from build123d import *

# Parameters (mm, degrees)
SKETCH1_W                 = 58.4
SKETCH1_H                 = 36.8
BOSS_EXTRUDE1_DEPTH       = 12.7
SKETCH2_R                 = 0.5
SKETCH2_R_2               = 0.75
SKETCH2_R_3               = 0.25
BOSS_EXTRUDE2_DEPTH       = 4.3
M3X0_5_TAPPED_HOLE1_D     = 2.5
M3X0_5_TAPPED_HOLE1_DEPTH = 4.5
M3X0_5_TAPPED_HOLE1_TIP   = 0.751075774
SKETCH6_R                 = 1.5
BOSS_EXTRUDE3_DEPTH       = 0.01


with BuildPart() as part:
    # Sketch1 → Boss-Extrude1 (new body)
    with BuildSketch(Plane(origin=(0, 0, 0), x_dir=(1, 0, 0), z_dir=(0, 1, 0))):
        Rectangle(SKETCH1_W, SKETCH1_H)
    extrude(amount=BOSS_EXTRUDE1_DEPTH)

    # Sketch2 → Boss-Extrude2 (add)
    with BuildSketch(Plane.XZ):
        with Locations((-25.4, 0)):
            Circle(SKETCH2_R)
        with Locations((-25.4, 3.81)):
            Circle(SKETCH2_R)
        with Locations((-25.4, 7.62)):
            Circle(SKETCH2_R)
        with Locations((-25.4, -7.62)):
            Circle(SKETCH2_R)
        with Locations((25.4, 7.62)):
            Circle(SKETCH2_R_2)
        with Locations((25.4, 3.81)):
            Circle(SKETCH2_R)
        with Locations((25.4, 0)):
            Circle(SKETCH2_R)
        with Locations((25.4, -3.81)):
            Circle(SKETCH2_R)
        with Locations((25.4, -7.62)):
            Circle(SKETCH2_R_2)
        with Locations((27.94, 0)):
            Circle(SKETCH2_R_3)
        with Locations((27.94, -2)):
            Circle(SKETCH2_R_3)
        with Locations((27.94, -4)):
            Circle(SKETCH2_R_3)
        with Locations((27.94, -6)):
            Circle(SKETCH2_R_3)
        with Locations((27.94, 2)):
            Circle(SKETCH2_R_3)
        with Locations((27.94, 4)):
            Circle(SKETCH2_R_3)
        with Locations((27.94, 6)):
            Circle(SKETCH2_R_3)
    extrude(amount=BOSS_EXTRUDE2_DEPTH)

    # M3x0.5 Tapped Hole1
    with Locations(Plane(origin=(-23.6, 12.7, -13.06), x_dir=(0, 0, 1), z_dir=(0, 1, 0))):
        with Locations((0, 0), (26.16, 0), (26.16, 47.24)):
            Hole(M3X0_5_TAPPED_HOLE1_D / 2, depth=M3X0_5_TAPPED_HOLE1_DEPTH)
            with Locations((0, 0, -(M3X0_5_TAPPED_HOLE1_DEPTH + M3X0_5_TAPPED_HOLE1_TIP / 2))):  # 118° drill point
                Cone(0, M3X0_5_TAPPED_HOLE1_D / 2, M3X0_5_TAPPED_HOLE1_TIP, mode=Mode.SUBTRACT)

    # Sketch6 → Boss-Extrude3 (add)
    with BuildSketch(Plane(origin=(0, 12.7, 0), x_dir=(1, 0, 0), z_dir=(0, 1, 0))):
        with Locations((8.9, -10.9)):
            Circle(SKETCH6_R)
    extrude(amount=BOSS_EXTRUDE3_DEPTH)


solid = part.part
CAD build for the part. Positions are in the model's coordinates, mm. A direction names the side the tool comes from. Round coordinates to 2 decimals unless told otherwise and drop trailing zeros. Write each loop counter-clockwise with the first axis right and the second up, starting at its lowest first coordinate (ties: lowest second). Pieces come first, ordered by that corner, then holes.
(1) Slice it at C-C, the plane x = 0. Write the cut outline in (y, z), and give its area (3 significant figures).
(2) Drop flat-ended pins along their axis: P1, Ø11, axis at x = 11, z = -7.5, coming from the +Y side; P2, Ø2, axis at x = -23.6, z = 13.1, coming from the +Y side; P3, Ø1.5, axis at x = -21.5, z = 0.5, coming from the -Y side. Give the stop position or say it passes through.
(3) Slice it at A-A, the plane y = -2.5. Count the separate pieces of the cut face and the enclosed holes in it, and give its area (3 significant figures).
(4) 3-axis set-ups, long thin cutter, end or side, ignore diameter. For faces 4 (the face through (-22.546, 10.418, 12.428)), 5 (the face through (26.115, -2.12, 7.845)), 6 (the face through (25, -4.3, 8)): which of +Z, -Z, +X, -X, +Y, -Y reach the whole face in a straight line?
(5) Mould opens along X. For faces 1 (the face through (0, 6, -18.4)), 2 (the face through (-29.2, 6, 0)), 3 (the face through (-23.68, 7.58, -12.86)) say: pulls with the +X half, pulls with the -X half, needs draft (parallel to the pull), parting line crosses it, or undercut.
(6) Probe line 1 along X through (y, z) = (9.85, 13.1); line 2 along Z through (x, y) = (-23.6, 10.7); line 3 along X through (y, z) = (9.5, -13). List the from-to ranges inside material, lowest first.
From the geometry:
1. outline: (0, -18.4) - (12.7, -18.4) - (12.7, 18.4) - (0, 18.4) - close
1. area: 467 mm2
2. P1: stops at y = 12.7
2. P2: stops at y = 8.05
2. P3: stops at y = 0
3. separate pieces: 16
3. enclosed holes: 0
3. area: 10.4 mm2
4. face 4: +Y
4. face 5: -Y
4. face 6: +Z, -Z, +X, -X, -Y
5. face 1: needs draft
5. face 2: pulls with the -X half
5. face 3: undercut
6. line 1: x = -29.2 to -24.85, -22.35 to 22.39, 24.89 to 29.2
6. line 2: z = -18.4 to -14.31, -11.81 to 11.85, 14.35 to 18.4
6. line 3: x = -29.2 to -24.85, -22.35 to 29.2
